Check sheet for the modelled part. Datum: model origin and axes. Units: mm. Face numbers are marked on the shaded views. A direction names the side the tool comes from. Give positions to 0.01 mm unless a question says otherwise; leave off trailing zeros. Order: outer loops, then holes, each group sorted by start corner. A loop starts at its lowest first (then second) coordinate and runs counter-clockwise, first axis right, second up. Notation, with made-up numbers: (74.5, -37) -> (113.5, -37) arc R23 cw to (113.5, -12) -> close; hole circle Ø3 at (77, 29.5). An arc over 180 degrees is marked (long way). Answer in a Markdown table with one row per item. Add a question column.
(1) Go/stop test with flat-tipped pins: pin 1 (1.5 mm diameter, centred on y = -2.5, z = -17.5, fed in from +X); pin 2 (1.8 mm diameter, centred on x = 0, z = -19, fed in from +Y); pin 3 (12 mm diameter, centred on x = 5.5, z = -21, fed in from -Y). Record where each tip stops, or that it passes through.
(2) Cross-section at C-C (y = -8.75). Record the cut outline in (x, z), then the cut area to 3 significant figures.
(3) Cross-section at D-D (y = 4.75). Record the cut outline in (x, z).
(4) Set-up check for the marked faces 1 and 2: record each of +Z, -Z, +X, -X, +Y, -Y from which the full face is reachable in a straight line by a thin tool's end or side.
(5) Thickness scan on L1, parallel to Y at x = 0, z = -1; L2, parallel to Z at x = 3, y = -8.5; L3, parallel to Y at x = 2, z = -23.25. Record the ranges inside material, lowest first. Write a range as [from, to].
(6) Cross-section at B-B (z = -3.5). Record the cut outline in (x, y), then the cut area to 3 significant figures.
(7) Cross-section at A-A (x = 0). Record the cut outline in (y, z).
```python
from build123d import *

# Parameters (mm, degrees)
SKETCH1_R           = 12.5
BOSS_EXTRUDE1_DEPTH = 5
SKETCH2_R           = 6.5
BOSS_EXTRUDE2_DEPTH = 22
CUT_EXTRUDE1_DEPTH  = 22
CUT_EXTRUDE2_REACH  = 34.272
SKETCH4_R           = 1.5


with BuildPart() as part:
    # Sketch1 → Boss-Extrude1 (new body)
    with BuildSketch(Plane.XY):
        Circle(SKETCH1_R)
    extrude(amount=-BOSS_EXTRUDE1_DEPTH)

    # Sketch2 → Boss-Extrude2 (add)
    with BuildSketch(Plane(origin=(0, 0, -5), x_dir=(-1, 0, 0), z_dir=(0, 0, -1))):
        Circle(SKETCH2_R)
    extrude(amount=BOSS_EXTRUDE2_DEPTH)

    # Sketch3 → Cut-Extrude1 (cut)
    with BuildSketch(Plane(origin=(0, 0, -27), x_dir=(-1, 0, 0), z_dir=(0, 0, -1))):
        with BuildLine():
            Line((-1.766352173, -2.3), (1.766352173, -2.3))
            ThreePointArc((1.766352173, -2.3), (0, 2.9), (-1.766352173, -2.3))
        make_face()
    extrude(amount=-CUT_EXTRUDE1_DEPTH, mode=Mode.SUBTRACT)

    # Sketch4 → Cut-Extrude2 (cut, up to next)
    with BuildSketch(Plane.XY, mode=Mode.PRIVATE) as cut_extrude2_sk1:
        with Locations((-8.227241336, 4.75)):
            Circle(SKETCH4_R)
    cut_extrude2_tool1 = extrude(cut_extrude2_sk1.sketch, amount=-CUT_EXTRUDE2_REACH, mode=Mode.PRIVATE) & part.part
    # Sketch4 → Cut-Extrude2 (cut, up to next)
    with BuildSketch(Plane.XY, mode=Mode.PRIVATE) as cut_extrude2_sk2:
        with Locations((8.227241336, 4.75)):
            Circle(SKETCH4_R)
    cut_extrude2_tool2 = extrude(cut_extrude2_sk2.sketch, amount=-CUT_EXTRUDE2_REACH, mode=Mode.PRIVATE) & part.part
    # Sketch4 → Cut-Extrude2 (cut, up to next)
    with BuildSketch(Plane.XY, mode=Mode.PRIVATE) as cut_extrude2_sk3:
        with Locations((0, -9.5)):
            Circle(SKETCH4_R)
    cut_extrude2_tool3 = extrude(cut_extrude2_sk3.sketch, amount=-CUT_EXTRUDE2_REACH, mode=Mode.PRIVATE) & part.part
    add(cut_extrude2_tool1.solids().sort_by_distance((-8.227241, 4.75, 0))[0], mode=Mode.SUBTRACT)
    add(cut_extrude2_tool2.solids().sort_by_distance((8.227241, 4.75, 0))[0], mode=Mode.SUBTRACT)
    add(cut_extrude2_tool3.solids().sort_by_distance((0, -9.5, 0))[0], mode=Mode.SUBTRACT)


solid = part.part
```
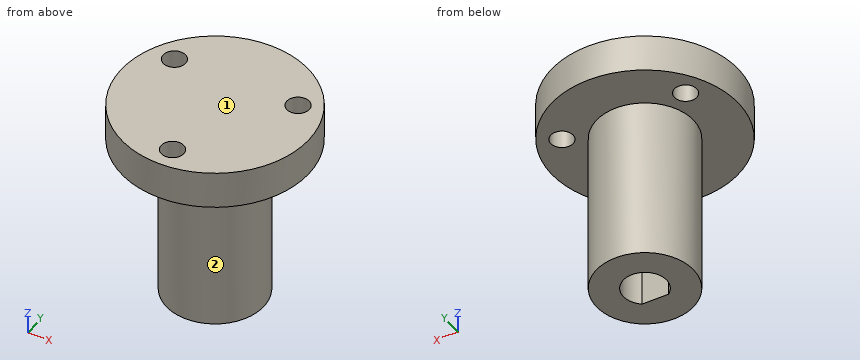
Answer below:
| question | item | result |
|---|---|---|
| 1 | pin 1 | stops at x = 6.26 |
| 1 | pin 2 | stops at y = 6.5 |
| 1 | pin 3 | stops at y = -6.5 |
| 2 | outline | (-8.93, -5) -> (-1.3, -5) -> (-1.3, 0) -> (-8.93, 0) -> close; (1.3, -5) -> (8.93, -5) -> (8.93, 0) -> (1.3, 0) -> close |
| 2 | area | 76.3 mm² |
| 3 | outline | (-11.56, -5) -> (-9.73, -5) -> (-9.73, 0) -> (-11.56, 0) -> close; (-6.73, -5) -> (-4.44, -5) -> (-4.44, -27) -> (4.44, -27) -> (4.44, -5) -> (6.73, -5) -> (6.73, 0) -> (-6.73, 0) -> close; (9.73, -5) -> (11.56, -5) -> (11.56, 0) -> (9.73, 0) -> close |
| 4 | face 1 | +Z, +X, -X, +Y, -Y |
| 4 | face 2 | -Z |
| 5 | L1 | y = [-12.5, -11], [-8, 12.5] |
| 5 | L2 | z = [-5, 0] |
| 5 | L3 | y = [-6.18, -2.1], [2.1, 6.18] |
| 6 | outline | circle Ø25 at (0, 0); hole circle Ø3 at (-8.23, 4.75); hole circle Ø3 at (0, -9.5); hole circle Ø3 at (8.23, 4.75) |
| 6 | area | 470 mm² |
| 7 | outline | (-12.5, -5) -> (-11, -5) -> (-11, 0) -> (-12.5, 0) -> close; (-8, -5) -> (-6.5, -5) -> (-6.5, -27) -> (-2.3, -27) -> (-2.3, -5) -> (2.9, -5) -> (2.9, -27) -> (6.5, -27) -> (6.5, -5) -> (12.5, -5) -> (12.5, 0) -> (-8, 0) -> close |
